from build123d import *

# Parameters (mm, degrees)
F0_W      = 72
F0_H      = 40
F1_DEPTH  = 16
F3_W      = 17
F3_H      = 9.5
F7_DEPTH  = 35
F4_W      = 12
F4_H      = 8
F8_DEPTH  = 20
F5_W      = 12
F5_H      = 8
F9_DEPTH  = 28
F6_W      = 18
F6_H      = 6
F10_DEPTH = 11
F11_R     = 3.25
F11_R_2   = 3
F12_DEPTH = 40.001
F13_W     = 6
F13_H     = 40
F13_W_2   = 5
F14_DEPTH = 8
F15_R     = 1
F16_R     = 4
F17_W     = 72
F17_H     = 10
F18_DEPTH = 16.001


with BuildPart() as f1:
    # F0 (on Top) → F1 (new body)
    with BuildSketch(Plane.XY):
        Rectangle(F0_W, F0_H)
    extrude(amount=F1_DEPTH)

    # F3 (on face) → F7 (cut)
    with BuildSketch(Plane.XZ.offset(20)):
        with Locations((-25, 8)):
            Rectangle(F3_W, F3_H)
    extrude(amount=-F7_DEPTH, mode=Mode.SUBTRACT)

    # F4 (on face) → F8 (cut)
    with BuildSketch(Plane.XZ.offset(20)):
        with Locations((-8, 8)):
            Rectangle(F4_W, F4_H)
    extrude(amount=-F8_DEPTH, mode=Mode.SUBTRACT)

    # F5 (on face) → F9 (cut)
    with BuildSketch(Plane.XZ.offset(20)):
        with Locations((6, 8)):
            Rectangle(F5_W, F5_H)
    extrude(amount=-F9_DEPTH, mode=Mode.SUBTRACT)

    # F6 (on face) → F10 (cut)
    with BuildSketch(Plane.XZ.offset(20)):
        with Locations((24.5, 8)):
            Rectangle(F6_W, F6_H)
    extrude(amount=-F10_DEPTH, mode=Mode.SUBTRACT)

    # F11 (on face) → F12 (cut, through all)
    with BuildSketch(Plane.XZ.offset(20)):
        with Locations((-25, 8)):
            Circle(F11_R)
        with Locations((-8, 8)):
            Circle(F11_R)
        with Locations((6, 8)):
            Circle(F11_R)
        with Locations((24.5, 8)):
            Circle(F11_R_2)
    extrude(amount=-F12_DEPTH, mode=Mode.SUBTRACT)

    # F13 (on face) → F14 (cut)
    with BuildSketch(Plane(origin=(0, 0, 0), x_dir=(1, 0, 0), z_dir=(0, 0, -1))):
        with Locations((-25, 0)):
            Rectangle(F13_W, F13_H)
        with Locations((-8, 0)):
            Rectangle(F13_W, F13_H)
        with Locations((6, 0)):
            Rectangle(F13_W, F13_H)
        with Locations((24.5, 0)):
            Rectangle(F13_W_2, F13_H)
    extrude(amount=-F14_DEPTH, mode=Mode.SUBTRACT)

    # F15
    f15_edges = [f1.edges().sort_by_distance(p)[0] for p in [
        (33.5, -14.5, 5),
        (33.5, -14.5, 11),
        (12, -6, 12),
        (-2, -10, 12),
        (-16.5, -2.5, 12.75),
        (-33.5, -2.5, 3.25),
        (-14, -10, 4),
        (0, -6, 4),
        (15.5, -14.5, 5),
        (15.5, -14.5, 11),
        (0, -6, 12),
        (-14, -10, 12),
        (-33.5, -2.5, 12.75),
        (12, -6, 4),
        (-2, -10, 4),
        (-16.5, -2.5, 3.25),
        (22, 0, 0),
        (27, 0, 0),
        (3, 0, 0),
        (9, 0, 0),
        (-11, 0, 0),
        (-5, 0, 0),
        (-28, 0, 0),
        (-22, 0, 0),
    ]]
    fillet(f15_edges, radius=F15_R)

    # F16
    f16_edges = [f1.edges().sort_by_distance(p)[0] for p in [
        (36, 0, 0),
        (36, 0, 16),
        (-36, 0, 0),
        (-36, 0, 16),
    ]]
    fillet(f16_edges, radius=F16_R)

    # F17 (on Top) → F18 (intersect, through all)
    with BuildSketch(Plane.XY):
        with Locations((0, -15)):
            Rectangle(F17_W, F17_H)
    extrude(amount=F18_DEPTH, mode=Mode.INTERSECT)


solid = f1.part
Build history of the part. All positions in model axes, mm. A direction names the side the tool comes from. Round coordinates to 2 decimals unless told otherwise and drop trailing zeros. Write each loop counter-clockwise with the first axis right and the second up, starting at its lowest first coordinate (ties: lowest second). Pieces come first, ordered by that corner, then holes. Notation, with made-up numbers: (13, 20) - (20, 20) arc R29 ccw to (20, 42) - close; hole circle Ø3 at (89.25, -36.5). An arc over 180 degrees is marked (long way). One line per question, with ' | ' between items.
1. Band-saw the part on B-B, the plane x = 29. Write the cut outline in (y, z), and give its area (3 significant figures).
Results are:
outline: (-20, 0) - (-10, 0) - (-10, 5) - (-20, 5) - close; (-20, 11) - (-10, 11) - (-10, 16) - (-20, 16) - close | area: 100 mm^2
2. Drill centre lines: line 1 along X through (y, z) = (-15, 7); line 2 along X through (y, z) = (-16.5, 3.75); line 3 along Z through (x, y) = (21.5, -10.25). Where is each one in solid material? Low to high. Write a range as from..to.
Results are:
line 1: -36..-33.5, -16.5..-14, -2..0, 12..15.5, 33.5..36 | line 2: -35.99..-33.37, -16.63..-11, -5..3, 9..22, 27..35.99 | line 3: 0.13..5, 11..16
3. Band-saw the part on A-A, the plane z = 8.25. Write the cut outline in (x, y).
Results are:
outline: (-36, -20) - (-33.5, -20) - (-33.5, -10) - (-36, -10) - close; (-16.5, -20) - (-14, -20) - (-14, -10) - (-16.5, -10) - close; (-2, -20) - (0, -20) - (0, -10) - (-2, -10) - close; (12, -20) - (15.5, -20) - (15.5, -10) - (12, -10) - close; (33.5, -20) - (36, -20) - (36, -10) - (33.5, -10) - close
4. Band-saw the part on D-D, the plane x = -26. Write the cut outline in (y, z).
Results are:
outline: (-20, 12.75) - (-10, 12.75) - (-10, 16) - (-20, 16) - close
5. Tool access for faces 4 (the face through (-1, -10, 10)), 5 (the face through (-22, -15, 2)), 6 (the face through (10, -15, 4)): list every direction of +Z, -Z, +X, -X, +Y, -Y with a clear straight run to the whole face (end or side of a thin tool).
Results are:
face 4: +Z, -Z, +X, -X, +Y | face 5: -Z, +Y, -Y | face 6: +Y, -Y
6. Mould opens along Z. For faces 1 (the face through (34.797, -14.93, 1.141)), 2 (the face through (36, -15, 8)), 3 (the face through (-4, -15, 4)) say: released by +Z, released by -Z, zero draft, split by the parting line, or undercut.
Results are:
face 1: released by -Z | face 2: zero draft | face 3: undercut
7. Drop flat-ended pins along their axis: pin 1 Ø1.1 at (y, z) = (-13.5, 2) entering from -X; pin 2 Ø1.5 at (y, z) = (-15.5, 3) entering from +X; pin 3 Ø3 at (x, y) = (-25, -13) entering from -Z. Give the stop position or say it passes through.
Results are:
pin 1: x = -35.73 | pin 2: x = 35.99 | pin 3: z = 12.75
8. Band-saw the part on C-C, the plane z = 2.5. Write the cut outline in (x, y).
Results are:
outline: (-35.71, -20) - (-28, -20) - (-28, -10) - (-35.71, -10) - close; (-22, -20) - (-11, -20) - (-11, -10) - (-22, -10) - close; (-5, -20) - (3, -20) - (3, -10) - (-5, -10) - close; (9, -20) - (22, -20) - (22, -10) - (9, -10) - close; (27, -20) - (35.71, -20) - (35.71, -10) - (27, -10) - close
